Build history of the part. All positions in model axes, mm. Give positions to 0.01 mm unless a question says otherwise; leave off trailing zeros. Loops run counter-clockwise (first coordinate to the right, second up) from the corner with the lowest first, then second, coordinate; pieces in that order, holes last. Notation, with made-up numbers: (-39.75, -5) - (18.25, -5) arc R34 ccw to (18.25, 32) - close; hole circle Ø1 at (-15, 82). An arc over 180 degrees is marked (long way). Return JSON: item names as keys, results as strings. Group by question number.
1) Drill centre lines: probe 1 along Y at (x, z) = (1, 1.4); probe 2 along X at (y, z) = (17, 0.9); probe 3 along Y at (x, z) = (-3.5, 0.9). Where is each one in solid material? Low to high. Write a range as from..to.
2) Slice it at A-A (x = 0). List the corners of the cut face in (y, z), and give its area (3 significant figures).
3) Slice it at C-C (z = 0.5). Count the separate pieces of the cut face and the enclosed holes in it, and give its area (3 significant figures).
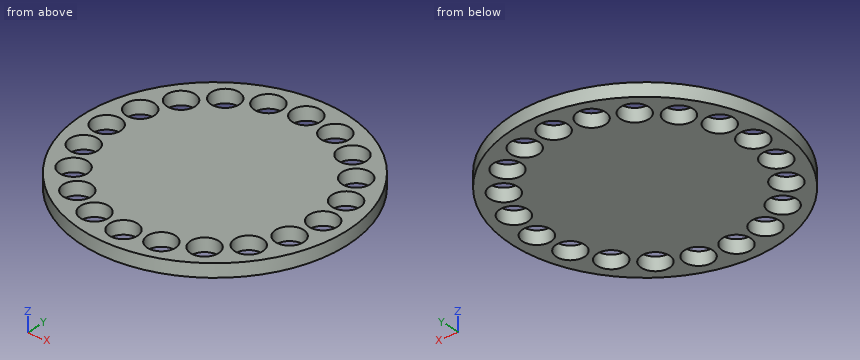
Autodesk Inventor part; units mm, degrees
ref_plane "YZ Plane" through (0, 0, 0) normal (1, 0, 0) x (0, 1, 0)
ref_plane "XZ Plane" through (0, 0, 0) normal (0, 1, 0) x (-1, 0, 0)
ref_plane "XY Plane" through (0, 0, 0) normal (0, 0, 1) x (1, 0, 0)
sketch "Skizze1" plane through (0, 0, 0) normal (0, 0, 1) x (1, 0, 0)
  circle A0 centre (0, 0) radius 20
  circle A1 centre (0, 16.4658) radius 2.1227
  circle A2 centre (-5.0882, 15.6599) radius 2.1227
  circle A3 centre (-9.6784, 13.3211) radius 2.1227
  circle A4 centre (-13.3211, 9.6784) radius 2.1227
  circle A5 centre (-15.6599, 5.0882) radius 2.1227
  circle A6 centre (-16.4658, 0) radius 2.1227
  circle A7 centre (-15.6599, -5.0882) radius 2.1227
  circle A8 centre (-13.3211, -9.6784) radius 2.1227
  circle A9 centre (-9.6784, -13.3211) radius 2.1227
  circle A10 centre (-5.0882, -15.6599) radius 2.1227
  circle A11 centre (0, -16.4658) radius 2.1227
  circle A12 centre (5.0882, -15.6599) radius 2.1227
  circle A13 centre (9.6784, -13.3211) radius 2.1227
  circle A14 centre (13.3211, -9.6784) radius 2.1227
  circle A15 centre (15.6599, -5.0882) radius 2.1227
  circle A16 centre (16.4658, 0) radius 2.1227
  circle A17 centre (15.6599, 5.0882) radius 2.1227
  circle A18 centre (13.3211, 9.6784) radius 2.1227
  circle A19 centre (9.6784, 13.3211) radius 2.1227
  circle A20 centre (5.0882, 15.6599) radius 2.1227
  dimension "d0" = 40
  dimension "d3" = 360
extrude "Extrusion1" add sketch "Skizze1" along normal blind 2
properties part number "EncoderWheel"
Results:
{
 "1": {"probe 1": "-19.97..-18.34, -14.59..14.59, 18.34..19.97", "probe 2": "-10.54..-6.73, -3.44..-2.05, 2.05..3.44, 6.73..10.54", "probe 3": "-19.69..-17.07, -14.25..14.25, 17.07..19.69"},
 "2": {"outline": "(-20, 0) - (-18.59, 0) - (-18.59, 2) - (-20, 2) - close; (-14.34, 0) - (14.34, 0) - (14.34, 2) - (-14.34, 2) - close; (18.59, 0) - (20, 0) - (20, 2) - (18.59, 2) - close", "area": "63.0 mm2"},
 "3": {"separate pieces": "1", "enclosed holes": "20", "area": "974 mm2"}
}
